```python
from build123d import *

# Parameters (mm, degrees)
F1_DEPTH = 19.05
F4_DEPTH = 9.525
F6_DEPTH = 3.175


with BuildPart() as f1:
    # F0 (on Front) → F1 (new body)
    with BuildSketch(Plane.XZ):
        Polygon((-508.79375, 0), (0, 0), (508.79375, 0), (508.79375, 150.8125), (0, 577.85), (-508.79375, 150.8125), align=None)
        Polygon((0, 63.5), (-445.29375, 63.5), (-445.29375, 121.206816), (0, 494.947904), (445.29375, 121.206816), (445.29375, 63.5), align=None, mode=Mode.SUBTRACT)
    extrude(amount=F1_DEPTH)

    # F3 (on face) → F4 (cut)
    with BuildSketch(Plane.XZ.offset(19.05)):
        Polygon((457.99375, 50.8), (457.99375, 127.127953), (0, 511.528323), (-457.99375, 127.127953), (-457.99375, 50.8), align=None)
        Polygon((-445.29375, 63.5), (-445.29375, 121.206816), (0, 494.947904), (445.29375, 121.206816), (445.29375, 63.5), align=None, mode=Mode.SUBTRACT)
    extrude(amount=-F4_DEPTH, mode=Mode.SUBTRACT)

    # F5 (on face) → F6 (cut)
    with BuildSketch(Plane.XZ.offset(9.525)):
        Polygon((0, 511.528323), (-457.99375, 127.127953), (-457.99375, 50.8), (457.99375, 50.8), (457.99375, 127.127953), align=None)
        Polygon((0, 507.383218), (454.81875, 125.647669), (454.81875, 53.975), (-454.81875, 53.975), (-454.81875, 125.647669), align=None, mode=Mode.SUBTRACT)
    extrude(amount=-F6_DEPTH, mode=Mode.SUBTRACT)


solid = f1.part
```
Check sheet for the modelled part. Datum: model origin and axes. Units: mm. A direction names the side the tool comes from. Give positions to 0.01 mm unless a question says otherwise; leave off trailing zeros. Order: outer loops, then holes, each group sorted by start corner. A loop starts at its lowest first (then second) coordinate and runs counter-clockwise, first axis right, second up. Notation, with made-up numbers: M 73,51.5 L 120,51.5 A18 cw 120,75.5 Z; hole C -32,-31 d5. An arc over 180 degrees is marked long. Answer in a Markdown table with one row per item. Add a question column.
Q1. Thickness scan on L1, parallel to X at y = -2.5, z = 107; L2, parallel to Z at x = -359, y = -7 (3 decimals); L3, parallel to Z at x = 377, y = -8.5 (3 decimals). Record the ranges inside material, lowest first.
Q2. Gauge pin test, flat ends, axial feed: pin 1 Ø4 at (y, z) = (-15.5, 284) entering from -X; pin 2 Ø5 at (y, z) = (-5, 427) entering from -X; pin 3 Ø1.5 at (x, y) = (-152.5, -11) entering from +Z; pin 4 Ø3.5 at (x, y) = (-134.5, -7.5) entering from -Z. Record the tip position at first contact, or that the pin passes through.
Q3. Sectioned sample at B-B, the plane x = 121. Record the boundary of the cut face in (y, z) (3 decimals).
Q4. Access from +Z, -Z, +X, -X, +Y, -Y to the whole of each face (thin tool, end or side, straight path). Record for faces 1 (the flat face through (232.2, -12.79, 316.64)), 2 (the flat face through (-250.835, -9.392, 367.321)), 3 (the flat face through (-225.764, -4.696, 305.461)).
Q5. Release check for a two-part mould opening along Z. For faces 4 (the flat face through (508.794, -9, 74)), 5 (the flat face through (-7, -9, 0)), 6 (the flat face through (224.226, -7.96, 319.188)) record: released by +Z, released by -Z, zero draft, split by the parting line, or undercut.
Q6. Sectioned sample at A-A, the plane y = -15. Record the boundary of the cut face in (x, z), and give its area (3 significant figures).
Verdict:
| question | item | result |
|---|---|---|
| 1 | L1 | -508.79 to -445.29, 445.29 to 508.79 |
| 1 | L2 | 0 to 50.8, 53.975 to 63.5, 193.634 to 206.07, 210.215 to 276.536 |
| 1 | L3 | 0 to 50.8, 53.975 to 63.5, 178.527 to 190.962, 195.107 to 261.429 |
| 2 | pin 1 | x = -352.49 |
| 2 | pin 2 | x = -182.71 |
| 2 | pin 3 | z = 450.48 |
| 2 | pin 4 | z = 0 |
| 3 | outline | M -19.05,0 L 0,0 L 0,63.5 L -9.525,63.5 L -9.525,53.975 L -6.35,53.975 L -6.35,50.8 L -19.05,50.8 Z; M -19.05,409.971 L -6.35,409.971 L -6.35,405.826 L -9.525,405.826 L -9.525,393.391 L 0,393.391 L 0,476.293 L -19.05,476.293 Z |
| 4 | face 1 | -Y |
| 4 | face 2 | +Z, -X, +Y, -Y |
| 4 | face 3 | +Y, -Y |
| 5 | face 4 | zero draft |
| 5 | face 5 | released by -Z |
| 5 | face 6 | undercut |
| 6 | outline | M -508.79,0 L 508.79,0 L 508.79,150.81 L 0,577.85 L -508.79,150.81 Z; hole M -457.99,50.8 L 457.99,50.8 L 457.99,127.13 L 0,511.53 L -457.99,127.13 Z |
| 6 | area | 125,000 mm² |
